For this review, take the finished solid that the model builds, in its own axes (mm). Face numbers are marked on the shaded views. Coordinates: 2 decimals unless noted, no trailing zeros. Write each loop counter-clockwise with the first axis right and the second up, starting at its lowest first coordinate (ties: lowest second). Pieces come first, ordered by that corner, then holes. Notation, with made-up numbers: M 80.25,33 L 114.25,33 A20 ccw 114.25,64 Z; hole C 88.25,-8 d11. An arc over 180 degrees is marked long. One line per question, with ' | ' between items.
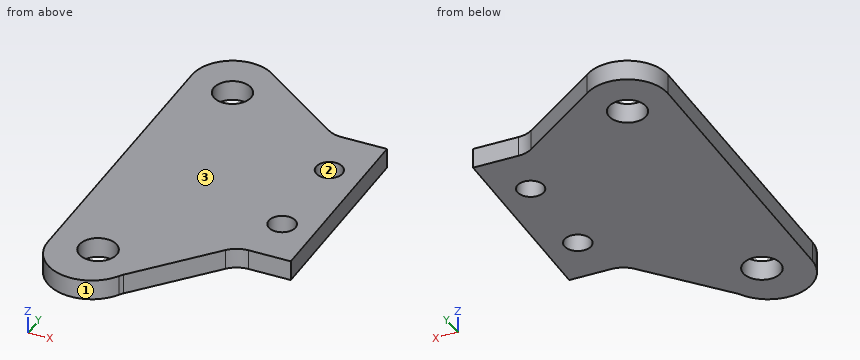
from build123d import *

# Parameters (mm, degrees)
F0_R     = 3.708309
F0_R_2   = 2.642108
F0_R_3   = 3.67947
F0_R_4   = 2.609813
F1_DEPTH = 4


with BuildPart() as f1:
    # F0 (on Top) → F1 (new body)
    with BuildSketch(Plane.XY):
        with BuildLine():
            Line((-21.411486, -22.898418), (-13.109211, -22.633235))
            Line((-13.109211, -22.633235), (-14.386204, 17.346376))
            Line((-14.386204, 17.346376), (-23.344903, 17.060226))
            ThreePointArc((-23.344903, 17.060226), (-24.884447, 17.251866), (-26.291138, 17.906195))
            Line((-26.291138, 17.906195), (-43.272432, 29.304598))
            ThreePointArc((-43.272432, 29.304598), (-51.794147, 30.076603), (-56.15294, 22.713415))
            Line((-56.15294, 22.713415), (-54.436188, -36.819749))
            ThreePointArc((-54.436188, -36.819749), (-47.787351, -45.022515), (-38.124586, -40.76536))
            ThreePointArc((-38.124586, -40.76536), (-37.887462, -40.377688), (-37.616119, -40.013148))
            Line((-37.616119, -40.013148), (-25.122912, -24.731226))
            ThreePointArc((-25.122912, -24.731226), (-23.465768, -23.412721), (-21.411486, -22.898418))
        make_face()
        with Locations((-45.345975, -34.922893)):
            Circle(F0_R, mode=Mode.SUBTRACT)
        with Locations((-19.947813, -12.667741)):
            Circle(F0_R_2, mode=Mode.SUBTRACT)
        with Locations((-47.129278, 20.936157)):
            Circle(F0_R_3, mode=Mode.SUBTRACT)
        with Locations((-20.412468, 6.623971)):
            Circle(F0_R_4, mode=Mode.SUBTRACT)
    extrude(amount=F1_DEPTH)


solid = f1.part
1. Clearance check with flat-ended pins moving along their axes: P1, Ø1, axis at y = -24, z = 2, coming from the -X side; P2, Ø1.5, axis at y = 17, z = 1, coming from the -X side; P3, Ø4.5, axis at x = -45.35, y = -34.92, coming from the +Z side; P4, Ø2, axis at y = 13, z = 1, coming from the +X side. State where each tip first meets the part, or that it passes through.
Computed values:
P1: stops at x = -54.82 | P2: stops at x = -56.01 | P3: passes through | P4: stops at x = -14.22
2. Draft analysis for pull direction Y (two halves, no side actions). For the marked faces 1, 2 and 3, state which applies: pulls with the +Y half, pulls with the -Y half, needs draft (parallel to the pull), parting line crosses it, or undercut.
Computed values:
face 1: pulls with the -Y half | face 2: undercut | face 3: needs draft
3. Take a section at A-A on y = 8.5. State the section outline as (x, z) points, plus the area to 3 significant figures.
Computed values:
outline: M -55.74,0 L -22.23,0 L -22.23,4 L -55.74,4 Z; M -18.6,0 L -14.1,0 L -14.1,4 L -18.6,4 Z | area: 152 mm2
4. Take a section at C-C on x = -46.5. State the section outline as (y, z) points.
Computed values:
outline: M -45.23,0 L -38.45,0 L -38.45,4 L -45.23,4 Z; M -31.4,0 L 17.31,0 L 17.31,4 L -31.4,4 Z; M 24.56,0 L 30.79,0 L 30.79,4 L 24.56,4 Z
5. For line 1 along Y through (x, z) = (-20.5, 1.3); line 2 along Y through (x, z) = (-46, 1.65); line 3 along X through (y, z) = (20.5, 1.1), list the stretches that pass through material, from the lowest coordinate up.
Computed values:
line 1: y = -22.87 to -15.25, -10.08 to 4.02, 9.23 to 17.15 | line 2: y = -45.26 to -38.57, -31.27 to 17.43, 24.44 to 30.66 | line 3: x = -56.09 to -50.78, -43.48 to -30.16
6. Take a section at D-D on y = -21. State the section outline as (x, z) points.
Computed values:
outline: M -54.89,0 L -13.16,0 L -13.16,4 L -54.89,4 Z
7. Take a section at B-B on z = 2.9. State the section outline as (x, y) points.
Computed values:
outline: M -56.15,22.71 L -54.44,-36.82 A8.7 ccw -38.12,-40.77 A5 cw -37.62,-40.01 L -25.12,-24.73 A5 cw -21.41,-22.9 L -13.11,-22.63 L -14.39,17.35 L -23.34,17.06 A5 cw -26.29,17.91 L -43.27,29.3 A8.01 ccw Z; hole C -47.13,20.94 d7.36; hole C -45.35,-34.92 d7.42; hole C -20.41,6.62 d5.22; hole C -19.95,-12.67 d5.28
